```python
from build123d import *

# Parameters (mm, degrees)
CROQUIS1_W              = 80
CROQUIS1_H              = 50
SALIENTE_EXTRUIR1_DEPTH = 12
CROQUIS2_R              = 2
CORTAR_EXTRUIR1_DEPTH   = 3
CROQUIS3_W              = 80
CROQUIS3_H              = 40
SALIENTE_EXTRUIR2_DEPTH = 500
CROQUIS4_W              = 60
CROQUIS4_H              = 500
CORTAR_EXTRUIR2_DEPTH   = 30
CROQUIS5_W              = 500
CROQUIS5_H              = 4
CORTAR_EXTRUIR3_DEPTH   = 1
CROQUIS6_W              = 500
CROQUIS6_H              = 4
CORTAR_EXTRUIR4_DEPTH   = 1
CROQUIS7_R              = 4
CORTAR_EXTRUIR5_DEPTH   = 621


with BuildPart() as part:
    # Croquis1 → Saliente-Extruir1 (new body)
    with BuildSketch(Plane.XY):
        Rectangle(CROQUIS1_W, CROQUIS1_H)
    saliente_extruir1 = extrude(amount=SALIENTE_EXTRUIR1_DEPTH)

    # Croquis2 → Cortar-Extruir1 (cut)
    with BuildSketch(Plane(origin=(0, 25, 0), x_dir=(1, 0, 0), z_dir=(0, 1, 0))):
        with Locations((-10, -6)):
            Circle(CROQUIS2_R)
        with Locations((10, -6)):
            Circle(CROQUIS2_R)
    cortar_extruir1 = extrude(amount=-CORTAR_EXTRUIR1_DEPTH, mode=Mode.SUBTRACT)

    # Croquis3 → Saliente-Extruir2 (add)
    with BuildSketch(Plane(origin=(0, 0, 0), x_dir=(-1, 0, 0), z_dir=(0, 0, -1))):
        with Locations((0, -5)):
            Rectangle(CROQUIS3_W, CROQUIS3_H)
    extrude(amount=SALIENTE_EXTRUIR2_DEPTH)

    # Croquis4 → Cortar-Extruir2 (cut)
    with BuildSketch(Plane(origin=(0, 15, 0), x_dir=(1, 0, 0), z_dir=(0, 1, 0))):
        with Locations((0, 250)):
            Rectangle(CROQUIS4_W, CROQUIS4_H)
    extrude(amount=-CORTAR_EXTRUIR2_DEPTH, mode=Mode.SUBTRACT)

    # Croquis5 → Cortar-Extruir3 (cut)
    with BuildSketch(Plane.ZY.offset(40)):
        with Locations((-250, 3)):
            Rectangle(CROQUIS5_W, CROQUIS5_H)
        with Locations((-250, -13)):
            Rectangle(CROQUIS5_W, CROQUIS5_H)
    extrude(amount=-CORTAR_EXTRUIR3_DEPTH, mode=Mode.SUBTRACT)

    # Croquis6 → Cortar-Extruir4 (cut)
    with BuildSketch(Plane(origin=(40, 0, 0), x_dir=(0, 0, -1), z_dir=(1, 0, 0))):
        with Locations((250, 3)):
            Rectangle(CROQUIS6_W, CROQUIS6_H)
        with Locations((250, -13)):
            Rectangle(CROQUIS6_W, CROQUIS6_H)
    extrude(amount=-CORTAR_EXTRUIR4_DEPTH, mode=Mode.SUBTRACT)

    # Simetría1: Saliente-Extruir1, Cortar-Extruir1 across plane
    add(saliente_extruir1.mirror(Plane(origin=(0, 0, -250), x_dir=(1, 0, 0), z_dir=(0, 0, -1))))
    add(cortar_extruir1.mirror(Plane(origin=(0, 0, -250), x_dir=(1, 0, 0), z_dir=(0, 0, -1))), mode=Mode.SUBTRACT)

    # Croquis7 → Cortar-Extruir5 (cut)
    with BuildSketch(Plane(origin=(0, 0, -512), x_dir=(-1, 0, 0), z_dir=(0, 0, -1))):
        with Locations((0, 10)):
            Circle(CROQUIS7_R)
    extrude(amount=-CORTAR_EXTRUIR5_DEPTH, mode=Mode.SUBTRACT)


solid = part.part
```
CAD build for the part. Positions are in the model's coordinates, mm. A direction names the side the tool comes from. Round coordinates to 2 decimals unless told otherwise and drop trailing zeros. Loops run counter-clockwise (first coordinate to the right, second up) from the corner with the lowest first, then second, coordinate; pieces in that order, holes last. Notation, with made-up numbers: M 54,81.25 L 104,81.25 A18 cw 104,105.25 Z; hole C -17.5,75 d10. An arc over 180 degrees is marked long. Return JSON: item names as keys, results as strings. Group by question number.
(1) Tool access for faces 1 (the flat face through (35, 15, -246)), 2 (the flat face through (30, 0, -247)), 3 (the flat face through (-1, 0, -512)): list every direction of +Z, -Z, +X, -X, +Y, -Y with a clear straight run to the whole face (end or side of a thin tool).
(2) Mould opens along X. For faces 4 (the flat face through (-1, 5, -500)), 5 (the flat face through (-1, 25, -506)), 6 (the flat face through (-40, -6, -246)) say: +X half, -X half, draft (parallel to the pull), parting line (faces both ways), or undercut.
(3) Saw through at A-A, the plane z = -329.5. List the corners of the cut face in (x, y), and give its area (3 significant figures).
(4) Saw through at B-B, the plane x = -21. List the corners of the cut face in (y, z), and give its area (3 significant figures).
(5) Drop flat-ended pins along their axis: P1, Ø3, axis at x = -36.5, z = -188, coming from the +Y side; P2, Ø5, axis at x = 11.5, z = -103.5, coming from the +Y side; P3, Ø2, axis at x = 9.5, z = 5.5, coming from the +Y side. Give the stop position or say it passes through.
(6) Wall check: probe 1 along Z at (x, y) = (10, 22.8); probe 2 along X at (y, z) = (23.2, 6); probe 3 along Z at (x, y) = (24, 10.5). Give the ranges that are in metal, low to high. Write a range as [from, to].
Answer list:
{
 "1": {"face 1": "+X, -X, +Y", "face 2": "+Y", "face 3": "-Z, +X, -X, +Y, -Y"},
 "2": {"face 4": "undercut", "face 5": "draft", "face 6": "-X half"},
 "3": {"outline": "M -40,-25 L 40,-25 L 40,-15 L 39,-15 L 39,-11 L 40,-11 L 40,1 L 39,1 L 39,5 L 40,5 L 40,15 L 30,15 L 30,-15 L -30,-15 L -30,15 L -40,15 L -40,5 L -39,5 L -39,1 L -40,1 L -40,-11 L -39,-11 L -39,-15 L -40,-15 Z", "area": "1,380 mm2"},
 "4": {"outline": "M -25,-512 L 25,-512 L 25,-500 L -15,-500 L -15,0 L 25,0 L 25,12 L -25,12 Z", "area": "6,200 mm2"},
 "5": {"P1": "y = 15", "P2": "y = -15", "P3": "y = 22"},
 "6": {"probe 1": "[-512, -508], [-504, -500], [0, 4], [8, 12]", "probe 2": "[-40, -12], [-8, 8], [12, 40]", "probe 3": "[-512, -500], [0, 12]"}
}
